```python
from build123d import *

# Parameters (mm, degrees)
F1_DEPTH = 20
F2_T     = -2
F3_W     = 50
F3_H     = 18
F4_DEPTH = 600
F5_W     = 30
F5_H     = 18
F6_DEPTH = 2


with BuildPart() as f1:
    # F0 (on Top) → F1 (new body)
    with BuildSketch(Plane.XY):
        with BuildLine():
            Line((945, 0), (0, 0))
            Line((0, 0), (0, -150))
            Line((0, -150), (1075, -150))
            Line((1075, -150), (1075, -130))
            ThreePointArc((1075, -130), (1036.923882, -38.076118), (945, 0))
        make_face()
    extrude(amount=F1_DEPTH)

    # F2
    f2_openings = [f1.faces().sort_by_distance(p)[0] for p in [
        (525.800735, -76.057549, 0),
    ]]
    offset(amount=F2_T, openings=f2_openings)

    # F3 (on face) → F4 (cut)
    with BuildSketch(Plane.XZ.offset(150)):
        with Locations((825, 9)):
            Rectangle(F3_W, F3_H)
    extrude(amount=-F4_DEPTH, mode=Mode.SUBTRACT)

    # F5 (on face) → F6 (cut)
    with BuildSketch(Plane.XZ.offset(150)):
        with Locations((1060, 9)):
            Rectangle(F5_W, F5_H)
    extrude(amount=-F6_DEPTH, mode=Mode.SUBTRACT)


solid = f1.part
```
Input: part model. Units: mm. Frame: model coordinates. A direction names the side the tool comes from. Coordinates: 2 decimals unless noted, no trailing zeros. Write each loop counter-clockwise with the first axis right and the second up, starting at its lowest first coordinate (ties: lowest second). Pieces come first, ordered by that corner, then holes.
1) Pin query (flat end, axial travel): pin 1 Ø8 at (x, y) = (745, -70.5) entering from -Z; pin 2 Ø4 at (y, z) = (-113, 10.5) entering from +X; pin 3 Ø9 at (y, z) = (-101.5, 5.5) entering from +X. Return the tip coordinate at first contact, or that it passes through.
2) Material intervals for line 1 along Y through (x, z) = (684.5, 13.5); line 2 along Z through (x, y) = (765.5, -140); line 3 along X through (y, z) = (-99.5, 17.5), sorted ascending.
3) Section C-C on y = -22. Output: boundary loops of the cut face in (x, z).
4) Set-up query: faces 1 (the flat face through (1073, -139, 9)), 2 (the flat face through (1075, -140, 10)), 3 (the flat face through (407, -2, 9)). Return all of +Z, -Z, +X, -X, +Y, -Y with unobstructed straight access to the full face (end or side cutting, diameter ignored); none if empty.
5) Section A-A on z = 13. Output: boundary loops of the cut face in (x, y).
6) Mould query, pull axis Y, two halves, no side actions, for faces 4 (the flat face through (479, 0, 10)), 5 (the flat face through (898, -2, 9)), 6 (the flat face through (0, -74, 10)). Classes: pulls with the +Y half, pulls with the -Y half, needs draft (parallel to the pull), parting line crosses it, or undercut.
7) Section B-B on x = 426. Output: boundary loops of the cut face in (y, z), and give its area (3 significant figures).
Check result:
1. pin 1: stops at z = 18
1. pin 2: stops at x = 1074.13
1. pin 3: stops at x = 1072.77
2. line 1: y = -150 to -148, -2 to 0
2. line 2: z = 18 to 20
2. line 3: x = 0 to 2, 1069.31 to 1071.37
3. outline: (0, 0) - (2, 0) - (2, 18) - (1013.7, 18) - (1013.7, 0) - (1017.36, 0) - (1017.36, 20) - (0, 20) - close
4. face 1: -Z, -Y
4. face 2: +Z, -Z, +X, +Y, -Y
4. face 3: -Z
5. outline: (0, -150) - (800, -150) - (800, -148) - (2, -148) - (2, -2) - (800, -2) - (800, 0) - (0, 0) - close; (850, -150) - (1045, -150) - (1045, -148) - (850, -148) - close; (850, -2) - (945, -2) arc R128 cw to (1073, -130) - (1073, -148) - (1075, -148) - (1075, -130) arc R130 ccw to (945, 0) - (850, 0) - close
6. face 4: pulls with the +Y half
6. face 5: undercut
6. face 6: needs draft
7. outline: (-150, 0) - (-148, 0) - (-148, 18) - (-2, 18) - (-2, 0) - (0, 0) - (0, 20) - (-150, 20) - close
7. area: 372 mm2
